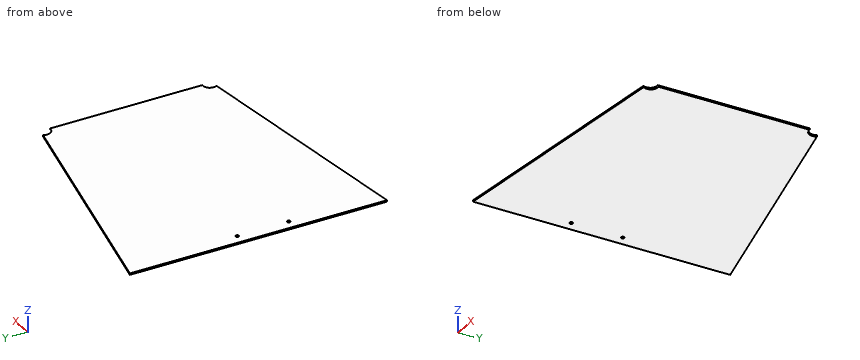
```python
from build123d import *

# Parameters (mm, degrees)
BOSS_EXTRUDE1_DEPTH = 3.175
SKETCH2_R           = 14.2875
CUT_EXTRUDE1_DEPTH  = 837.34562622
CUT_EXTRUDE2_DEPTH  = 880.199971547
SKETCH4_R           = 3.175
CUT_EXTRUDE3_DEPTH  = 870.180090301


with BuildPart() as part:
    # Sketch1 → Boss-Extrude1 (new body)
    with BuildSketch(Plane(origin=(1.950344864, 0, -26.264644174), x_dir=(-0.9972542674746705, 0, -0.07405353471346578), z_dir=(0.07405353471346578, 0, -0.9972542674746705))):
        Polygon((-183.644373355, -298.45), (-183.644373355, 298.45), (-826.760197391, 177.8), (-826.760197391, -177.8), align=None)
    extrude(amount=BOSS_EXTRUDE1_DEPTH)

    # Sketch2 → Cut-Extrude1 (cut, through all)
    with BuildSketch(Plane(origin=(825.5, 212.942802273, 150.983020837), x_dir=(1, 0, 0), z_dir=(0, 0.32191156150474026, 0.9467697431633416))):
        Circle(SKETCH2_R)
    cut_extrude1 = extrude(amount=-CUT_EXTRUDE1_DEPTH, mode=Mode.SUBTRACT)

    # Mirror1: Cut-Extrude1 across plane
    add(cut_extrude1.mirror(Plane.ZX), mode=Mode.SUBTRACT)

    # Sketch3 → Cut-Extrude2 (cut, through all)
    with BuildSketch(Plane(origin=(1.950344864, 0, -26.264644174), x_dir=(0.9972542674746705, 0, 0.0740535347134658), z_dir=(-0.0740535347134658, 0, 0.9972542674746706))):
        Polygon((348.744373355, -267.476862261), (348.744373355, 267.476862261), (183.644373355, 298.45), (183.644373355, -298.45), align=None)
    extrude(amount=-CUT_EXTRUDE2_DEPTH, mode=Mode.SUBTRACT)

    # Sketch4 → Cut-Extrude3 (cut, through all)
    with BuildSketch(Plane(origin=(2.185464837, 0, -29.430926473), x_dir=(-0.9972542674746705, 0, -0.0740535347134658), z_dir=(0.0740535347134658, 0, -0.9972542674746706))):
        with Locations((-367.794373355, 33)):
            Circle(SKETCH4_R)
        with Locations((-367.794373355, -74)):
            Circle(SKETCH4_R)
    extrude(amount=-CUT_EXTRUDE3_DEPTH, mode=Mode.SUBTRACT)


solid = part.part
```
The model under review builds one solid part; all positions refer to its coordinate system, in mm. Round coordinates to 2 decimals unless told otherwise and drop trailing zeros. Order: outer loops, then holes, each group sorted by start corner. A loop starts at its lowest first (then second) coordinate and runs counter-clockwise, first axis right, second up. Notation, with made-up numbers: M 7.25,46 L 57.25,46 A27 ccw 57.25,71 Z; hole C 59.25,65.25 d11. An arc over 180 degrees is marked long. Use a Markdown table: item, result.
1) Consider section B-B (x = 776.5). Write out the cut boundary in (y, z), then the cut area to 3 significant figures.
Report:
| item | result |
|---|---|
| outline | M -187.24,28.07 L 187.24,28.07 L 187.19,31.25 L -187.19,31.25 Z |
| area | 1,190 mm^2 |
2) Insertion check: pin 1 (4 mm diameter, centred on x = 730.5, z = 22.5, fed in from -Y); pin 2 (1.5 mm diameter, centred on x = 679.5, z = 21, fed in from +Y); pin 3 (2 mm diameter, centred on x = 764, y = 150.5, fed in from -Z); pin 4 (12 mm diameter, centred on x = 496, y = -70, fed in from -Z). Each pin has a flat end and moves straight along its axis. Give the tip position at first contact, or say it passes through.
Report:
| item | result |
|---|---|
| pin 1 | through |
| pin 2 | y = 205.63 |
| pin 3 | z = 27.07 |
| pin 4 | z = 6.79 |
3) Consider section A-A (y = 43.5). Write out the cut boundary in (x, z).
Report:
| item | result |
|---|---|
| outline | M 349.74,-0.44 L 349.97,-3.61 L 826.68,31.79 L 826.44,34.96 Z |
4) Wall thickness on line 1 along Z through (x, y) = (562, 159); line 2 along Y through (x, z) = (762, 27.5); line 3 along Z through (x, y) = (462, 108): over which ranges is each line inside the solid? List them lowest first. Write a range as [from, to].
Report:
| item | result |
|---|---|
| line 1 | [12.14, 15.32] |
| line 2 | [-189.96, 189.96] |
| line 3 | [4.71, 7.9] |
